Model file for the job. Use its own axes, mm. A direction names the side the tool comes from. Round coordinates to 2 decimals unless told otherwise and drop trailing zeros. Loops run counter-clockwise (first coordinate to the right, second up) from the corner with the lowest first, then second, coordinate; pieces in that order, holes last. Notation, with made-up numbers: (34, -37.75) -> (61, -37.75) arc R33 ccw to (61, -1.75) -> close; hole circle Ø6 at (81, 67.5). An arc over 180 degrees is marked (long way). Use a Markdown table: item, result.
Autodesk Inventor part; units mm, degrees
ref_plane "YZ Plane" through (0, 0, 0) normal (1, 0, 0) x (0, 1, 0)
ref_plane "XZ Plane" through (0, 0, 0) normal (0, 1, 0) x (-1, 0, 0)
ref_plane "XY Plane" through (0, 0, 0) normal (0, 0, 1) x (1, 0, 0)
sketch "Sketch1" plane through (0, 0, 0) normal (0, 0, 1) x (1, 0, 0)
  line L0 (15, -10) -> (-15, -10)
  line L1 (-15, -10) -> (-15, 10)
  line L2 (-15, 10) -> (15, 10)
  line L3 (15, 10) -> (15, -10)
  line L4 (15, -10) -> (-15, 10) construction
  line L5 (-15, -10) -> (15, 10) construction
  line L6 (20, -15) -> (-20, -15)
  line L7 (-20, -15) -> (-20, 15)
  line L8 (-20, 15) -> (20, 15)
  line L9 (20, 15) -> (20, -15)
  line L10 (20, -15) -> (-20, 15) construction
  line L11 (-20, -15) -> (20, 15) construction
  point P0 (0, 0)
  dimension "d0" = 30
  dimension "d1" = 20
  dimension "d2" = 40
  dimension "d3" = 30
extrude "Extrusion1" add sketch "Sketch1" along normal blind 15
fillet "Fillet1" radius 1 4 edges at (-15, -10, 7.5) (-15, 10, 7.5) (15, 10, 7.5) (15, -10, 7.5)
fillet "Fillet2" radius 1 4 edges at (-20, 15, 7.5) (-20, -15, 7.5) (20, 15, 7.5) (20, -15, 7.5)
properties part number "agarose-mold-mouse-brain"
Q1. Band-saw the part on B-B, the plane z = 3. Give the cut face in (x, y).
Results list:
| item | result |
|---|---|
| outline | (-20, -14) arc R1 ccw to (-19, -15) -> (19, -15) arc R1 ccw to (20, -14) -> (20, 14) arc R1 ccw to (19, 15) -> (-19, 15) arc R1 ccw to (-20, 14) -> close; hole (-15, -9) arc R1 ccw to (-14, -10) -> (14, -10) arc R1 ccw to (15, -9) -> (15, 9) arc R1 ccw to (14, 10) -> (-14, 10) arc R1 ccw to (-15, 9) -> close |
Q2. Drill centre lines: L1, parallel to Y at x = 11.5, z = 13; L2, parallel to X at y = 1.5, z = 5.5. Where is each one in solid material? Low to high. Write a range as from..to.
Results list:
| item | result |
|---|---|
| L1 | y = -15..-10, 10..15 |
| L2 | x = -20..-15, 15..20 |
Q3. Flat gauge pin, fed straight in: pin 1 (8 mm diameter, centred on x = 0.5, y = 3.5, fed in from -Z). Where does the tip first touch, or does it go through?
Results list:
| item | result |
|---|---|
| pin 1 | passes through |
Q4. Tool access for faces 1 (the face through (-19.699, 14.715, 7.605)), 2 (the face through (15, 0, 7)): list every direction of +Z, -Z, +X, -X, +Y, -Y with a clear straight run to the whole face (end or side of a thin tool).
Results list:
| item | result |
|---|---|
| face 1 | +Z, -Z, -X, +Y |
| face 2 | +Z, -Z |
Q5. Band-saw the part on A-A, the plane y = -8. Give the cut face in (x, z).
Results list:
| item | result |
|---|---|
| outline | (-20, 0) -> (-15, 0) -> (-15, 15) -> (-20, 15) -> close; (15, 0) -> (20, 0) -> (20, 15) -> (15, 15) -> close |
Q6. Pull direction X, two halves, no side cores. Call faces 3 (the face through (0, 10, 7)), 4 (the face through (0, -15, 7)), 5 (the face through (-15, 0, 7)), 6 (the face through (-20, 0, 7)): released by +X, released by -X, zero draft, split by the parting line, or undercut.
Results list:
| item | result |
|---|---|
| face 3 | undercut |
| face 4 | zero draft |
| face 5 | undercut |
| face 6 | released by -X |
Q7. Band-saw the part on C-C, the plane x = -5. Give the cut face in (y, z), plus the area to 3 significant figures.
Results list:
| item | result |
|---|---|
| outline | (-15, 0) -> (-10, 0) -> (-10, 15) -> (-15, 15) -> close; (10, 0) -> (15, 0) -> (15, 15) -> (10, 15) -> close |
| area | 150 mm² |
